Can you work these out from the model? Positions are in its coordinate system, mm. Coordinates: 2 decimals unless noted, no trailing zeros. Write each loop counter-clockwise with the first axis right and the second up, starting at its lowest first coordinate (ties: lowest second). Pieces come first, ordered by that corner, then holes.
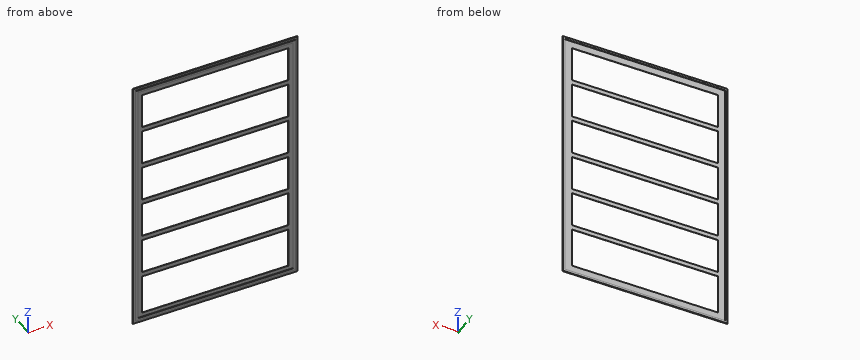
```python
from build123d import *

# Parameters (mm, degrees)
F0_W     = 72
F0_H     = 0.1
F1_DEPTH = 110
F2_W     = 69.8
F2_H     = 107.8
F2_W_2   = 67.8
F2_H_2   = 105.8
F3_DEPTH = 0.25
F4_W     = 72
F4_H     = 110
F4_W_2   = 70
F4_H_2   = 108
F5_DEPTH = 0.25
F6_W     = 63.8
F6_H     = 15
F6_H_2   = 17
F7_DEPTH = 2


with BuildPart() as f1:
    # F0 (on Top) → F1 (new body)
    with BuildSketch(Plane.XY):
        Rectangle(F0_W, F0_H)
    extrude(amount=F1_DEPTH)

    # F2 (on face) → F3 (join)
    with BuildSketch(Plane.XZ.offset(0.05)):
        with Locations((0, 55)):
            Rectangle(F2_W, F2_H)
        with Locations((0, 55)):
            Rectangle(F2_W_2, F2_H_2, mode=Mode.SUBTRACT)
    extrude(amount=F3_DEPTH)

    # F4 (on face) → F5 (join)
    with BuildSketch(Plane(origin=(0, 0.05, 0), x_dir=(-1, 0, 0), z_dir=(0, 1, 0))):
        with Locations((0, 55)):
            Rectangle(F4_W, F4_H)
        with Locations((0, 55)):
            Rectangle(F4_W_2, F4_H_2, mode=Mode.SUBTRACT)
    extrude(amount=F5_DEPTH)

    # F6 (on face) → F7 (cut)
    with BuildSketch(Plane.XZ.offset(0.05)):
        with Locations((0, 98.4)):
            Rectangle(F6_W, F6_H)
        with Locations((0, 81.4)):
            Rectangle(F6_W, F6_H)
        with Locations((0, 64.4)):
            Rectangle(F6_W, F6_H)
        with Locations((0, 47.4)):
            Rectangle(F6_W, F6_H)
        with Locations((0, 30.4)):
            Rectangle(F6_W, F6_H)
        with Locations((0, 12.4)):
            Rectangle(F6_W, F6_H_2)
    extrude(amount=-F7_DEPTH, mode=Mode.SUBTRACT)


solid = f1.part
```
1. If we section it at B-B, the plane y = -0.15: List the corners of the cut face in (x, z) for me, plus the area to 3 significant figures.
2. If I drill on L1, parallel to Z at x = 20.5, y = 0.15; L2, parallel to X at y = 0.1, z = 40; L3, parallel to X at y = 0, z = 102, over which ranges is the centre line in solid material (lowest first)?
3. If we section it at C-C, the plane x = -11: Count the separate pieces of the cut face and the enclosed holes in it, plus the area to 3 significant figures.
4. I'm going to push flat-ended pins straight in: P1, Ø8, axis at x = -1.5, z = 92.5, coming from the -Y side; P2, Ø8, axis at x = 23.5, z = 17.5, coming from the +Y side. Where does each tip first touch, or does it pass through?
5. If we section it at A-A, the plane z = 10.5: List the corners of the cut face in (x, y) for me.
Answers:
1. outline: (-34.9, 1.1) - (34.9, 1.1) - (34.9, 108.9) - (-34.9, 108.9) - close; hole (-33.9, 2.1) - (33.9, 2.1) - (33.9, 107.9) - (-33.9, 107.9) - close
1. area: 351 mm2
2. L1: z = 0 to 1, 109 to 110
2. L2: x = -36 to -35, 35 to 36
2. L3: x = -36 to -31.9, 31.9 to 36
3. separate pieces: 7
3. enclosed holes: 0
3. area: 2.80 mm2
4. P1: stops at y = -0.05
4. P2: stops at y = 0.05
5. outline: (-36, -0.05) - (-34.9, -0.05) - (-34.9, -0.3) - (-33.9, -0.3) - (-33.9, -0.05) - (-31.9, -0.05) - (-31.9, 0.05) - (-35, 0.05) - (-35, 0.3) - (-36, 0.3) - close; (31.9, -0.05) - (33.9, -0.05) - (33.9, -0.3) - (34.9, -0.3) - (34.9, -0.05) - (36, -0.05) - (36, 0.3) - (35, 0.3) - (35, 0.05) - (31.9, 0.05) - close
